from build123d import *

# Parameters (mm, degrees)
PAD_DEPTH       = 6.5
POCKET_DEPTH    = 6
SKETCH002_R     = 13.5
POCKET001_DEPTH = 1
SKETCH003_W     = 5.4
SKETCH003_H     = 6.5
PAD001_DEPTH    = 3.8
POCKET002_DEPTH = 10
SKETCH008_R     = 0.6
POCKET003_DEPTH = 2
SKETCH009_R     = 0.6
POCKET004_DEPTH = 2
FILLET_R        = 2.9
FILLET001_R     = 2.9
FILLET002_R     = 5
FILLET003_R     = 5
FILLET004_R     = 5
FILLET005_R     = 5
SKETCH010_W     = 3.95
SKETCH010_H     = 6.5
PAD002_DEPTH    = 4.5
POCKET005_DEPTH = 10
SKETCH012_R     = 0.6
POCKET006_DEPTH = 2
SKETCH013_R     = 0.6
POCKET007_DEPTH = 2
FILLET006_R     = 3.4
FILLET007_R     = 3.4
SKETCH014_R     = 20.45
SKETCH014_R_2   = 19.5
POCKET008_DEPTH = 0.3
SKETCH015_R     = 0.9
PAD003_DEPTH    = 6
FILLET008_R     = 1
POCKET009_DEPTH = 4
POCKET010_DEPTH = 4


with BuildPart() as part:
    # Sketch → Pad (new body)
    with BuildSketch(Plane.XY):
        with BuildLine():
            Line((-22.5019915649, 16), (-22.5019915649, -16))
            Line((-22.5019915649, -16), (-16.2858834578, -17.9))
            ThreePointArc((-16.2858834578, -17.9), (0.2206895736, -24.1989937004), (16.6096357576, -17.6))
            Line((16.6096357576, -17.6), (25.6083856708, -17.45))
            Line((25.6083856708, 17.45), (25.6083856708, -17.45))
            Line((16.6096357576, 17.6), (25.6083856708, 17.45))
            ThreePointArc((16.6096357576, 17.6), (0.2206895736, 24.1989937004), (-16.2858834578, 17.9))
            Line((-22.5019915649, 16), (-16.2858834578, 17.9))
        make_face()
    extrude(amount=PAD_DEPTH)

    # Sketch001 → Pocket (cut)
    with BuildSketch(Plane.XY):
        with BuildLine():
            Line((-14.8539557021, 16.9), (-21.2122180433, 15.55))
            Line((-21.2122180433, 15.55), (-21.2122180433, -15.55))
            Line((-21.2122180433, -15.55), (-14.8539557021, -16.9))
            ThreePointArc((-14.8539557021, -16.9), (-0.0760301383, -22.4998715423), (14.739402973, -17))
            Line((14.739402973, -17), (23.6191552218, -16.4))
            Line((23.6191552218, 16.4), (23.6191552218, -16.4))
            Line((14.739402973, 17), (23.6191552218, 16.4))
            ThreePointArc((14.739402973, 17), (-0.0760301383, 22.4998715423), (-14.8539557021, 16.9))
        make_face()
    extrude(amount=POCKET_DEPTH, mode=Mode.SUBTRACT)

    # Sketch002 (on Face19 of Pocket) → Pocket001 (cut)
    with BuildSketch(Plane(origin=(0, 0, 6), x_dir=(1, 0, 0), z_dir=(0, 0, -1))):
        Circle(SKETCH002_R)
    extrude(amount=-POCKET001_DEPTH, mode=Mode.SUBTRACT)

    # Sketch003 (on Face6 of Pocket001) → Pad001 (join)
    with BuildSketch(Plane.YZ.offset(25.6083856708)):
        with Locations((-14.75, 3.25)):
            Rectangle(SKETCH003_W, SKETCH003_H)
        with Locations((14.75, 3.25)):
            Rectangle(SKETCH003_W, SKETCH003_H)
    extrude(amount=PAD001_DEPTH)

    # Sketch006 → Pocket002 (cut)
    with BuildSketch(Plane.XY.offset(6.5)):
        with BuildLine():
            ThreePointArc((25.6083856708, 17.45), (27.3544703324, 16.0634214301), (29.4083856708, 15.1957558499))
            Line((29.4083856708, 17.45), (29.4083856708, 15.1957558499))
            Line((29.4083856708, 17.45), (25.6083856708, 17.45))
        make_face()
        with BuildLine():
            ThreePointArc((29.4083856708, -15.1957558499), (27.3544703324, -16.0634214301), (25.6083856708, -17.45))
            Line((29.4083856708, -17.45), (25.6083856708, -17.45))
            Line((29.4083856708, -15.1957558499), (29.4083856708, -17.45))
        make_face()
    extrude(amount=-POCKET002_DEPTH, mode=Mode.SUBTRACT)

    # Sketch008 (on Face27 of Pocket002) → Pocket003 (cut)
    with BuildSketch(Plane(origin=(0, -12.05, 0), x_dir=(-1, 0, 0), z_dir=(0, 1, 0))):
        with Locations((-27.7083856708, 1.7)):
            Circle(SKETCH008_R)
    extrude(amount=-POCKET003_DEPTH, mode=Mode.SUBTRACT)

    # Sketch009 (on Face26 of Pocket003) → Pocket004 (cut)
    with BuildSketch(Plane.XZ.offset(-12.05)):
        with Locations((27.7083856708, 1.7)):
            Circle(SKETCH009_R)
    extrude(amount=-POCKET004_DEPTH, mode=Mode.SUBTRACT)

    # Fillet
    fillet_edges = [part.edges().sort_by_distance(p)[0] for p in [
        (29.408386, -13.622878, 6.5),
    ]]
    fillet(fillet_edges, radius=FILLET_R)

    # Fillet001
    fillet001_edges = [part.edges().sort_by_distance(p)[0] for p in [
        (29.408386, 13.622878, 6.5),
    ]]
    fillet(fillet001_edges, radius=FILLET001_R)

    # Fillet002
    fillet002_edges = [part.edges().sort_by_distance(p)[0] for p in [
        (16.609636, -17.6, 3.25),
    ]]
    fillet(fillet002_edges, radius=FILLET002_R)

    # Fillet003
    fillet003_edges = [part.edges().sort_by_distance(p)[0] for p in [
        (16.609636, 17.6, 3.25),
    ]]
    fillet(fillet003_edges, radius=FILLET003_R)

    # Fillet004
    fillet004_edges = [part.edges().sort_by_distance(p)[0] for p in [
        (-16.285883, -17.9, 3.25),
    ]]
    fillet(fillet004_edges, radius=FILLET004_R)

    # Fillet005
    fillet005_edges = [part.edges().sort_by_distance(p)[0] for p in [
        (-16.285883, 17.9, 3.25),
    ]]
    fillet(fillet005_edges, radius=FILLET005_R)

    # Sketch010 (on Face4 of Fillet005) → Pad002 (join)
    with BuildSketch(Plane(origin=(-22.5019915649, 0, 0), x_dir=(0, -1, 0), z_dir=(-1, 0, 0))):
        with Locations((-14.025, 3.25)):
            Rectangle(SKETCH010_W, SKETCH010_H)
        with Locations((14.025, 3.25)):
            Rectangle(SKETCH010_W, SKETCH010_H)
    extrude(amount=PAD002_DEPTH)

    # Sketch011 (on Face6 of Pad002) → Pocket005 (cut)
    with BuildSketch(Plane.XY.offset(6.5)):
        with BuildLine():
            ThreePointArc((-27.0019915649, 14.6), (-24.6759937451, 15.0557212933), (-22.5019915649, 16))
            Line((-22.5019915649, 16), (-27.0019915649, 16))
            Line((-27.0019915649, 16), (-27.0019915649, 14.6))
        make_face()
        with BuildLine():
            ThreePointArc((-22.5019915649, -16), (-24.6759937451, -15.0557212933), (-27.0019915649, -14.6))
            Line((-27.0019915649, -14.6), (-27.0019915649, -16))
            Line((-27.0019915649, -16), (-22.5019915649, -16))
        make_face()
    extrude(amount=-POCKET005_DEPTH, mode=Mode.SUBTRACT)

    # Sketch012 (on Face23 of Pocket005) → Pocket006 (cut)
    with BuildSketch(Plane(origin=(0, -12.05, 0), x_dir=(-1, 0, 0), z_dir=(0, 1, 0))):
        with Locations((25.3019915649, 1.7)):
            Circle(SKETCH012_R)
    extrude(amount=-POCKET006_DEPTH, mode=Mode.SUBTRACT)

    # Sketch013 (on Face21 of Pocket006) → Pocket007 (cut)
    with BuildSketch(Plane.XZ.offset(-12.05)):
        with Locations((-25.3019915649, 1.7)):
            Circle(SKETCH013_R)
    extrude(amount=-POCKET007_DEPTH, mode=Mode.SUBTRACT)

    # Fillet006
    fillet006_edges = [part.edges().sort_by_distance(p)[0] for p in [
        (-27.001992, 13.325, 6.5),
    ]]
    fillet(fillet006_edges, radius=FILLET006_R)

    # Fillet007
    fillet007_edges = [part.edges().sort_by_distance(p)[0] for p in [
        (-27.001992, -13.325, 6.5),
    ]]
    fillet(fillet007_edges, radius=FILLET007_R)

    # Sketch014 (on Face4 of Fillet007) → Pocket008 (cut)
    with BuildSketch(Plane.XY.offset(6.5)):
        Circle(SKETCH014_R)
        Circle(SKETCH014_R_2, mode=Mode.SUBTRACT)
    extrude(amount=-POCKET008_DEPTH, mode=Mode.SUBTRACT)

    # Sketch015 (on Face55 of Pocket008) → Pad003 (join)
    with BuildSketch(Plane(origin=(0, 0, 6), x_dir=(1, 0, 0), z_dir=(0, 0, -1))):
        with Locations((-18.42, 13.32)):
            Circle(SKETCH015_R)
        with Locations((-18.42, -13.32)):
            Circle(SKETCH015_R)
        with Locations((7.27, 18.56)):
            Circle(SKETCH015_R)
        with Locations((5.37, -19.79)):
            Circle(SKETCH015_R)
    extrude(amount=PAD003_DEPTH)

    # Fillet008
    fillet008_edges = [part.edges().sort_by_distance(p)[0] for p in [
        (-19.32, -13.32, 6),
        (6.37, -18.56, 6),
        (-19.32, 13.32, 6),
        (4.47, 19.79, 6),
    ]]
    fillet(fillet008_edges, radius=FILLET008_R)

    # Sketch016 (on Face16 of Fillet008) → Pocket009 (cut)
    with BuildSketch(Plane(origin=(0, 0, 0), x_dir=(1, 0, 0), z_dir=(0, 0, -1))):
        with BuildLine():
            Line((-5, 23.6778377391), (-5, 21.9374109685))
            ThreePointArc((5, 21.9374109685), (0, 22.5), (-5, 21.9374109685))
            Line((5, 23.6778377391), (5, 21.9374109685))
            ThreePointArc((5, 23.6778377391), (0, 24.2), (-5, 23.6778377391))
        make_face()
    extrude(amount=-POCKET009_DEPTH, mode=Mode.SUBTRACT)

    # Sketch017 (on Face16 of Pocket009) → Pocket010 (cut)
    with BuildSketch(Plane(origin=(0, 0, 0), x_dir=(1, 0, 0), z_dir=(0, 0, -1))):
        with BuildLine():
            Line((-3.499984119, -22.2261132717), (-3.5, -23.9455632634))
            ThreePointArc((-3.5, -23.9455632634), (0, -24.2000019575), (3.5, -23.9455632634))
            Line((3.5000158811, -22.2261082701), (3.5, -23.9455632634))
            ThreePointArc((-3.499984119, -22.2261132717), (1.60767e-05, -22.5), (3.5000158811, -22.2261082701))
        make_face()
        with BuildLine():
            ThreePointArc((-13.9498796389, -17.6536358312), (-11.25, -19.4855715851), (-8.3135572795, -20.9077680626))
            Line((-8.3135572795, -20.9077680626), (-8.9416927184, -22.487466094))
            ThreePointArc((-15.0038705449, -18.987466094), (-12.1, -20.9578147716), (-8.9416927184, -22.487466094))
            Line((-13.9498796389, -17.6536358312), (-15.0038705449, -18.987466094))
        make_face()
        with BuildLine():
            ThreePointArc((8.3135572795, -20.9077680626), (11.25, -19.4855715851), (13.9498796389, -17.6536358312))
            Line((13.9498796389, -17.6536358312), (15.0038705449, -18.987466094))
            ThreePointArc((8.9416927184, -22.487466094), (12.1, -20.9578147716), (15.0038705449, -18.987466094))
            Line((8.3135572795, -20.9077680626), (8.9416927184, -22.487466094))
        make_face()
    extrude(amount=-POCKET010_DEPTH, mode=Mode.SUBTRACT)


solid = part.part
Work out the finished part from the listing and answer in its coordinate system (mm). A direction names the side the tool comes from. Give positions to 0.01 mm unless a question says otherwise; leave off trailing zeros. Write each loop counter-clockwise with the first axis right and the second up, starting at its lowest first coordinate (ties: lowest second). Pieces come first, ordered by that corner, then holes. Notation, with made-up numbers: (-35, 43) - (11, 43) arc R32 cw to (11, 82) - close; hole circle Ø8 at (-24.5, 47). An arc over 180 degrees is marked (long way). One line per item, written item: value. Start each with the question number.
1. Given pin 1 (1.6 mm diameter, centred on x = -25.3, z = 1.7, fed in from +Y); pin 2 (2.5 mm diameter, centred on x = 0, y = -23.5, fed in from -Z); pin 3 (1.9 mm diameter, centred on y = 23, z = 2, fed in from +X), each flat-ended and moving along its own axis, determine where each tip first touches the part or whether it passes through.
2. Find section C-C (z = 1.7). State how many separate pieces and enclosed holes the cut face has, then the cut area to 3 significant figures.
3. Consider probe 1 along Y at (x, z) = (0, 6.45); probe 2 along X at (y, z) = (-19, 2.75); probe 3 along X at (y, z) = (-7, 4.5). Determine where each line is inside the solid, lowest interval first.
4. For faces 1 (the flat face through (-25, 12.05, 3)), 2 (the flat face through (-14.47, 18.31, 1.97)), 3 (the flat face through (28, 14.05, 2)), 4 (the cylindrical face through (-14.37, 13.18, 6.35)), 5 (the flat face through (5, -23, 2)), determine the directions among +Z, -Z, +X, -X, +Y, -Y from which every point of the face is accessible in a straight line to the end or side of a thin tool.
5. Find section B-B (x = -10). Write down the section's boundary in (y, z).
6. Find section A-A (y = 0). Write down the section's boundary in (x, z).
7. Find section D-D (x = -18.42). Write down the section's boundary in (y, z).
8. For a pull along X with two mould halves and no side action, classify faces 6 (the cylindrical face through (-0.3, -22.5, 4.3)), 7 (the flat face through (-27.002, 13, 2)), 8 (the flat face through (0, -23, 4)), 9 (the flat face through (-18, -13, 0)) as +X half, -X half, draft (parallel to the pull), parting line (faces both ways), or undercut.
Geometry results:
1. pin 1: y = 15.11
1. pin 2: z = 4
1. pin 3: x = 8.94
2. separate pieces: 8
2. enclosed holes: 0
2. area: 262 mm2
3. probe 1: -24.2 to -20.45, -19.5 to -13.5, 13.5 to 19.5, 20.45 to 24.2
3. probe 2: -14.99 to -12.05, 6.48 to 8.06, 12.05 to 14.99
3. probe 3: -22.5 to -21.21, 23.62 to 25.61
4. face 1: +Z, -Z, -X
4. face 2: -Z, +Y
4. face 3: none
4. face 4: +Z
4. face 5: -Z, -Y
5. outline: (-22.04, 0) - (-20.16, 0) - (-20.16, 6) - (-9.07, 6) - (-9.07, 6.5) - (-16.74, 6.5) - (-16.74, 6.2) - (-17.84, 6.2) - (-17.84, 6.5) - (-22.04, 6.5) - close; (9.07, 6) - (20.16, 6) - (20.16, 4) - (22.04, 4) - (22.04, 6.5) - (17.84, 6.5) - (17.84, 6.2) - (16.74, 6.2) - (16.74, 6.5) - (9.07, 6.5) - close
6. outline: (-22.5, 0) - (-21.21, 0) - (-21.21, 6) - (-13.5, 6) - (-13.5, 6.5) - (-19.5, 6.5) - (-19.5, 6.2) - (-20.45, 6.2) - (-20.45, 6.5) - (-22.5, 6.5) - close; (13.5, 6) - (23.62, 6) - (23.62, 0) - (25.61, 0) - (25.61, 6.5) - (20.45, 6.5) - (20.45, 6.2) - (19.5, 6.2) - (19.5, 6.5) - (13.5, 6.5) - close
7. outline: (-17.25, 0) - (-16.14, 0) - (-16.14, 6) - (-15.22, 6) arc R1 cw to (-14.22, 5) - (-14.22, 0) - (-12.42, 0) - (-12.42, 5) arc R1 cw to (-11.42, 6) - (11.42, 6) arc R1 cw to (12.42, 5) - (12.42, 0) - (14.22, 0) - (14.22, 5) arc R1 cw to (15.22, 6) - (16.14, 6) - (16.14, 0) - (17.25, 0) - (17.25, 6.5) - (8.88, 6.5) - (8.88, 6.2) - (6.4, 6.2) - (6.4, 6.5) - (-6.4, 6.5) - (-6.4, 6.2) - (-8.88, 6.2) - (-8.88, 6.5) - (-17.25, 6.5) - close
8. face 6: undercut
8. face 7: -X half
8. face 8: undercut
8. face 9: draft
